Autodesk Inventor part; units mm, degrees
ref_plane "Arbeitsebene1" through (0, 0, 0) normal (0, 0, -1) x (-1, 0, 0)
ref_plane "Arbeitsebene4" through (0, 0, 0) normal (0, 0, -1) x (-1, 0, 0)
ref_plane "Arbeitsebene3" through (-15, 100, 0) normal (0, 1, 0) x (1, 0, 0)
ref_plane "Arbeitsebene1" through (0, 0, 0) normal (0, 0, -1) x (-1, 0, 0)
sketch "Skizze3" plane through (0, 0, 0) normal (0, 0, -1) x (-1, 0, 0)
  point P0 (0, 0)
ref_plane "Arbeitsebene4" through (0, 0, 0) normal (0, 0, -1) x (-1, 0, 0)
sketch "Skizze4" plane through (0, 0, 0) normal (0, 0, -1) x (-1, 0, 0)
  line L0 (15, 68) -> (-15, 68)
  line L1 (-15, 68) -> (-15, 60)
  line L2 (-15, 60) -> (15, 60)
  line L3 (15, 60) -> (15, 68)
  line L4 (-15, 76) -> (15, 76)
  line L5 (15, 76) -> (15, 84)
  line L6 (15, 84) -> (-15, 84)
  line L7 (-15, 84) -> (-15, 76)
  line L8 (-15, 92) -> (15, 92)
  line L9 (15, 92) -> (15, 100)
  line L10 (15, 100) -> (-15, 100)
  line L11 (-15, 100) -> (-15, 92)
  point P0 (0, 0)
  dimension "d7" = 30
  dimension "d8" = 8
  dimension "d9" = 30
  dimension "d10" = 8
  dimension "d11" = 8
extrude "Extrusion3" add sketch "Skizze4" along normal blind 60
ref_plane "Arbeitsebene3" through (-15, 100, 0) normal (0, 1, 0) x (1, 0, 0)
sketch "Skizze5" plane through (-15, 100, 0) normal (0, 1, 0) x (1, 0, 0)
  circle A0 centre (15, 30) radius 7
  line L0 (0, 60) -> (30, 60)
  arc A1 (30, 60) -> (0, 60) centre (15, 60) ccw
  point P0 (15, 0)
  dimension "d14" = 14
  dimension "d15" = 15
extrude "Extrusion4" cut sketch "Skizze5" against normal blind 40 contours A0
sketch "Skizze6" plane through (0, 0, -60) normal (0, 0, -1) x (-1, 0, 0)
  circle A0 centre (0, 80) radius 90
  point P0 (0, 0)
  point P1 (-15, 76)
  dimension "d19" = 180
extrude "Extrusion5" add sketch "Skizze6" along normal blind 30
fillet "Rundung1" radius 2 2 edges at (90, 80, -90) (90, 80, -60)
sketch "Skizze8" plane through (0, 80, -90) normal (0, 0, -1) x (-1, 0, 0)
  point P0 (0, -80)
properties part number "Press_Stempel"
Work out the finished part from the listing and answer in its coordinate system (mm). A direction names the side the tool comes from. Round coordinates to 2 decimals unless told otherwise and drop trailing zeros. Write each loop counter-clockwise with the first axis right and the second up, starting at its lowest first coordinate (ties: lowest second). Pieces come first, ordered by that corner, then holes. Notation, with made-up numbers: (12.25, 32) -> (59.25, 32) arc R15 cw to (59.25, 47) -> close; hole circle Ø5 at (65, -18.5). An arc over 180 degrees is marked (long way). Write each question's results on one line, items separated by ' | '.
Q1. Section A-A, the plane z = -49.5 is taken. Write down the section's boundary in (x, y), then the cut area to 3 significant figures.
Data:
outline: (-15, 60) -> (15, 60) -> (15, 68) -> (-15, 68) -> close; (-15, 76) -> (15, 76) -> (15, 84) -> (-15, 84) -> close; (-15, 92) -> (15, 92) -> (15, 100) -> (-15, 100) -> close | area: 720 mm^2
Q2. Section C-C, the plane z = -30 is taken. Write down the section's boundary in (x, y), then the cut area to 3 significant figures.
Data:
outline: (-15, 60) -> (-7, 60) -> (-7, 68) -> (-15, 68) -> close; (-15, 76) -> (-7, 76) -> (-7, 84) -> (-15, 84) -> close; (-15, 92) -> (-7, 92) -> (-7, 100) -> (-15, 100) -> close; (7, 60) -> (15, 60) -> (15, 68) -> (7, 68) -> close; (7, 76) -> (15, 76) -> (15, 84) -> (7, 84) -> close; (7, 92) -> (15, 92) -> (15, 100) -> (7, 100) -> close | area: 384 mm^2
Q3. Which of the six approach directions +Z, -Z, +X, -X, +Y, -Y give full straight-line access (tool end or side, diameter ignored) to faces 5 (the cylindrical face through (-85.844, 52.966, -74.818)), 6 (the cylindrical face through (-1.517, 80.056, -23.166)), 7 (the flat face through (-15, 64, -30)), 8 (the flat face through (15, 96, -30)), 9 (the flat face through (4, 92, -23))?
Data:
face 5: +Z, -Z | face 6: +Y, -Y | face 7: +Z, -X, +Y, -Y | face 8: +Z, +X, +Y, -Y | face 9: +Z, +X, -X
Q4. Straight lines are drawn through the part: line 1 along Y through (x, z) = (-3, -56.5); line 2 along X through (y, z) = (63, -30); line 3 along Z through (x, y) = (0, 77). For each, find the intervals that lie inside material, in ascending order. Write a range as [from, to].
Data:
line 1: [60, 68], [76, 84], [92, 100] | line 2: [-15, -7], [7, 15] | line 3: [-90, -37], [-23, 0]
Q5. Section B-B, the plane y = 80 is taken. Write down the section's boundary in (x, z), then the cut area to 3 significant figures.
Data:
outline: (-90, -88) arc R2 ccw to (-88, -90) -> (88, -90) arc R2 ccw to (90, -88) -> (90, -62) arc R2 ccw to (88, -60) -> (15, -60) -> (15, 0) -> (-15, 0) -> (-15, -60) -> (-88, -60) arc R2 ccw to (-90, -62) -> close; hole circle Ø14 at (0, -30) | area: 7,040 mm^2
Q6. Determine the mould class of faces 1 (the flat face through (4, 76, -23)), 2 (the flat face through (-4, 68, -23)), 3 (the flat face through (-4, 100, -23)), 4 (the flat face through (1, 81, -90)) for opening direction Y: released by +Y, released by -Y, zero draft, split by the parting line, or undercut.
Data:
face 1: undercut | face 2: undercut | face 3: released by +Y | face 4: zero draft
Q7. Flat-ended cylindrical pins translate along their axes: P1, Ø24, axis at x = -0.5, z = -29, coming from the -Y side; P2, Ø15, axis at x = 1.5, z = -26.5, coming from the +Y side; P3, Ø6.5, axis at y = 94, z = -24.5, coming from the -X side; P4, Ø8, axis at x = 67, y = 12, coming from the -Z side. Find the tip coordinate at first contact, or state that the pin passes through.
Data:
P1: y = 60 | P2: y = 100 | P3: x = -15 | P4: through
Q8. Section D-D, the plane x = 0 is taken. Give the number of separate pieces and of enclosed holes in the cut face, then the cut area to 3 significant figures.
Data:
separate pieces: 4 | enclosed holes: 0 | area: 6,500 mm^2
